```python
from build123d import *

# Parameters (mm, degrees)
SKETCH1_R           = 3.175
SKETCH1_R_2         = 3.2639
SKETCH1_R_3         = 1.55
SKETCH1_R_4         = 11.43
BOSS_EXTRUDE1_DEPTH = 4.7625
CUT_EXTRUDE1_DEPTH  = 322.291260875


with BuildPart() as part:
    # Sketch1 → Boss-Extrude1 (new body)
    with BuildSketch(Plane.XY):
        with BuildLine():
            Line((-260.35, 0), (-260.35, -3.2004))
            ThreePointArc((-260.35, -3.2004), (-258.497567548, -7.672567548), (-254.0254, -9.525))
            Line((-254.0254, -9.525), (-190.4746, -9.525))
            ThreePointArc((-190.4746, -9.525), (-186.002432452, -7.672567548), (-184.15, -3.2004))
            Line((-184.15, -3.2004), (-184.15, 0))
            ThreePointArc((-184.15, 0), (-170.132415912, 70.47115407), (-130.213713756, 130.213713756))
            Line((-130.213713756, 130.213713756), (-127.950689213, 132.476738298))
            ThreePointArc((-127.950689213, 132.476738298), (-126.098256761, 136.948905846), (-127.950689213, 141.421073395))
            Line((-127.950689213, 141.421073395), (-172.887890843, 186.358275024))
            ThreePointArc((-172.887890843, 186.358275024), (-177.360058391, 188.210707476), (-181.832225939, 186.358275024))
            Line((-181.832225939, 186.358275024), (-183.161638698, 185.028862266))
            ThreePointArc((-183.161638698, 185.028862266), (-184.195780986, 184.338914621), (-185.415571777, 184.098938684))
            Line((-185.415571777, 184.098938684), (-203.140946764, 184.148452962))
            ThreePointArc((-203.140946764, 184.148452962), (-217.580337842, 180.720298054), (-228.884291539, 171.104223407))
            Line((-228.884291539, 171.104223407), (-232.899485557, 165.597414859))
            ThreePointArc((-232.899485557, 165.597414859), (-238.444512868, 152.777545082), (-237.951278447, 138.818565579))
            Line((-237.951278447, 138.818565579), (-235.302655594, 128.744521776))
            ThreePointArc((-235.302655594, 128.744521776), (-234.372087536, 117.99517122), (-237.095069858, 107.554871341))
            ThreePointArc((-237.095069858, 107.554871341), (-254.469864559, 55.020092069), (-260.35, 0))
        make_face()
        with Locations(Location((-158.649272178, 111.08741631, 0), (0, 0, 180))):
            Circle(SKETCH1_R, mode=Mode.SUBTRACT)
        with Locations(Location((-148.363657521, 124.491890306, 0), (0, 0, 180))):
            Circle(SKETCH1_R, mode=Mode.SUBTRACT)
        with Locations(Location((-136.948905846, 136.948905846, 0), (0, 0, 180))):
            Circle(SKETCH1_R, mode=Mode.SUBTRACT)
        with Locations(Location((-227.895302491, 17.935749283, 0), (0, 0, 180))):
            Circle(SKETCH1_R_2, mode=Mode.SUBTRACT)
        with Locations(Location((-222.283763803, 53.365610177, 0), (0, 0, 180))):
            Circle(SKETCH1_R_2, mode=Mode.SUBTRACT)
        with Locations(Location((-211.198861132, 87.481432639, 0), (0, 0, 180))):
            Circle(SKETCH1_R_2, mode=Mode.SUBTRACT)
        with Locations(Location((-194.913541571, 119.443171894, 0), (0, 0, 180))):
            Circle(SKETCH1_R_2, mode=Mode.SUBTRACT)
        with Locations(Location((-173.828803736, 148.463823848, 0), (0, 0, 180))):
            Circle(SKETCH1_R_2, mode=Mode.SUBTRACT)
        with Locations(Location((-215.499095978, 171.127431131, 0), (0, 0, 180))):
            Circle(SKETCH1_R_3, mode=Mode.SUBTRACT)
        with Locations(Location((-201.499096038, 157.127431191, 0), (0, 0, 180))):
            Circle(SKETCH1_R_3, mode=Mode.SUBTRACT)
        with Locations(Location((-215.499095978, 143.127431251, 0), (0, 0, 180))):
            Circle(SKETCH1_R_3, mode=Mode.SUBTRACT)
        with Locations(Location((-229.499095918, 157.127431191, 0), (0, 0, 180))):
            Circle(SKETCH1_R_3, mode=Mode.SUBTRACT)
        with Locations(Location((-215.499095978, 157.127431191, 0), (0, 0, 180))):
            Circle(SKETCH1_R_4, mode=Mode.SUBTRACT)
        with Locations(Location((-254, 0, 0), (0, 0, 180))):
            Circle(SKETCH1_R_2, mode=Mode.SUBTRACT)
        with Locations(Location((-250.872838511, 39.73435412, 0), (0, 0, 180))):
            Circle(SKETCH1_R_2, mode=Mode.SUBTRACT)
        with Locations(Location((-241.568355139, 78.490316571, 0), (0, 0, 180))):
            Circle(SKETCH1_R_2, mode=Mode.SUBTRACT)
        with Locations(Location((-226.315657144, 115.313586934, 0), (0, 0, 180))):
            Circle(SKETCH1_R_2, mode=Mode.SUBTRACT)
        with Locations(Location((-179.605122421, 179.605122421, 0), (0, 0, 180))):
            Circle(SKETCH1_R_2, mode=Mode.SUBTRACT)
    extrude(amount=BOSS_EXTRUDE1_DEPTH)

    # Sketch2 → Cut-Extrude1 (cut, through all)
    with BuildSketch(Plane.XY.offset(4.7625)):
        with BuildLine():
            Line((-202.692, -9.525), (-183.642, -9.525))
            Line((-183.642, -9.525), (-183.642, 9.525))
            ThreePointArc((-183.642, 9.525), (-189.221615818, -3.945384182), (-202.692, -9.525))
        make_face()
    extrude(amount=-CUT_EXTRUDE1_DEPTH, mode=Mode.SUBTRACT)


solid = part.part
```
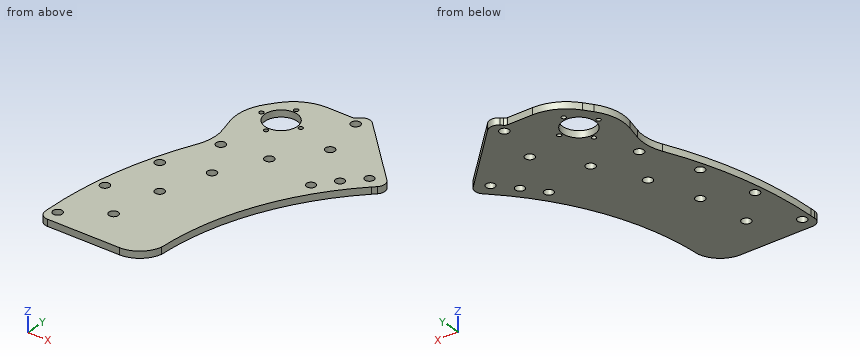
Here's how the part is built. I have some questions about the finished solid (model axes, mm). Give positions to 0.01 mm unless a question says otherwise; leave off trailing zeros. Order: outer loops, then holes, each group sorted by start corner. A loop starts at its lowest first (then second) coordinate and runs counter-clockwise, first axis right, second up. Notation, with made-up numbers: (64.5, 76.25) - (96.5, 76.25) arc R26 cw to (96.5, 92.25) - close; hole circle Ø2 at (27.25, 32.25). An arc over 180 degrees is marked (long way). Answer as a JSON object with one key per item and string values. Group by question number.
Item 1: Please list where these lines run through material, in increasing order: probe 1 along X at (y, z) = (180.5, 2.95); probe 2 along Y at (x, z) = (-204, 1.15) (3 decimals); probe 3 along Y at (x, z) = (-194, 2.85).
Item 2: If we section it at A-A on y = 73: Please give me the cut outline in (x, z), and give its area (3 significant figures).
Item 3: For P1, Ø8.5, axis at x = -211.2, y = 87.48, coming from the -Z side; P2, Ø6, axis at x = -227.9, y = 17.94, coming from the +Z side; P3, Ø1, axis at x = -204.5, z = 2, coming from the +Y side; P4, Ø1.5, axis at y = 144, z = 4, coming from the -X side, each with a flat end and sliding along its axis, tell me the tip position at first contact or that it passes through.
Item 4: If we section it at B-B on z = 1.7: Give the number of separate pieces and of enclosed holes in the cut face, and give its area (3 significant figures).
Result set:
{
 "1": {"probe 1": "-218.01 to -182.74, -176.47 to -167.03", "probe 2": "-9.525 to 184.139", "probe 3": "-7.43 to 116.31, 122.58 to 184.12"},
 "2": {"outline": "(-249.91, 0) - (-169.06, 0) - (-169.06, 4.76) - (-249.91, 4.76) - close", "area": "385 mm²"},
 "3": {"P1": "z = 0", "P2": "through", "P3": "y = 184.14", "P4": "x = -238.92"},
 "4": {"separate pieces": "1", "enclosed holes": "18", "area": "15,300 mm²"}
}
